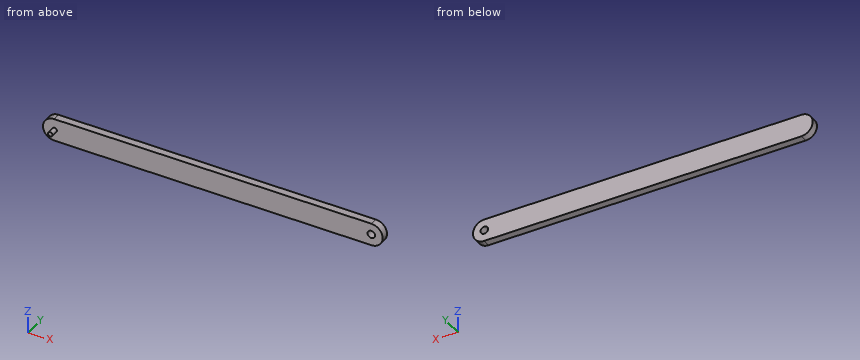
from build123d import *

# Parameters (mm, degrees)
SKETCH1_W           = 114.3
SKETCH1_H           = 7.62
BOSS_EXTRUDE1_DEPTH = 2.54
FILLET1_RADIUS      = 3.81
FILLET1_LENGTH      = 2.54
FILLET4_RADIUS      = 3.81
FILLET4_LENGTH      = 2.54
SKETCH4_R           = 1.27
CUT_EXTRUDE1_DEPTH  = 2.54
SKETCH6_R           = 0.762
BOSS_EXTRUDE3_DEPTH = 2.54


with BuildPart() as part:
    # Sketch1 → Boss-Extrude1 (new body)
    with BuildSketch(Plane(origin=(0, 0, 0), x_dir=(1, 0, 0), z_dir=(0, 1, 0))):
        Rectangle(SKETCH1_W, SKETCH1_H)
    extrude(amount=BOSS_EXTRUDE1_DEPTH)

    # Fillet1: full round fillet: the end face becomes a half cylinder, R = half its width
    fillet1_face = Plane((57.15, 1.27, 0), x_dir=(0, -1, 0), z_dir=(1, 0, 0))  # on the end face: x along it, z out of the body
    fillet1_slab = fillet1_face.offset(-FILLET1_RADIUS / 2) * Box(FILLET1_LENGTH, 2 * FILLET1_RADIUS, FILLET1_RADIUS, mode=Mode.PRIVATE)  # the body's end, R deep
    fillet1_round = Plane((53.34, 1.27, 0), x_dir=(1, 0, 0), z_dir=(0, -1, 0)) * Cylinder(FILLET1_RADIUS, FILLET1_LENGTH, mode=Mode.PRIVATE)  # its axis R under the face
    add(fillet1_slab - fillet1_round, mode=Mode.SUBTRACT)

    # Fillet4: full round fillet: the end face becomes a half cylinder, R = half its width
    fillet4_face = Plane((-57.15, 1.27, 0), x_dir=(0, 1, 0), z_dir=(-1, 0, 0))  # on the end face: x along it, z out of the body
    fillet4_slab = fillet4_face.offset(-FILLET4_RADIUS / 2) * Box(FILLET4_LENGTH, 2 * FILLET4_RADIUS, FILLET4_RADIUS, mode=Mode.PRIVATE)  # the body's end, R deep
    fillet4_round = Plane((-53.34, 1.27, 0), x_dir=(-1, 0, 0), z_dir=(0, 1, 0)) * Cylinder(FILLET4_RADIUS, FILLET4_LENGTH, mode=Mode.PRIVATE)  # its axis R under the face
    add(fillet4_slab - fillet4_round, mode=Mode.SUBTRACT)

    # Sketch4 → Cut-Extrude1 (cut)
    with BuildSketch(Plane(origin=(0, 0, 0), x_dir=(-1, 0, 0), z_dir=(0, -1, 0))):
        with Locations(Location((-53.34, 0, 0), (0, 0, 90))):
            Circle(SKETCH4_R)
    extrude(amount=-CUT_EXTRUDE1_DEPTH, mode=Mode.SUBTRACT)

    # Sketch6 → Boss-Extrude3 (add)
    with BuildSketch(Plane(origin=(0, 0, 0), x_dir=(-1, 0, 0), z_dir=(0, -1, 0))):
        with Locations(Location((53.234546108, 0, 0), (0, 0, 90))):
            Circle(SKETCH6_R)
    extrude(amount=BOSS_EXTRUDE3_DEPTH)


solid = part.part
The listing builds one solid part. Answer for the finished solid, in the listing's coordinates (mm). Coordinates: 2 decimals unless noted, no trailing zeros. Write each loop counter-clockwise with the first axis right and the second up, starting at its lowest first coordinate (ties: lowest second). Pieces come first, ordered by that corner, then holes. Notation, with made-up numbers: M 68,21.25 L 87,21.25 A14 ccw 87,28.25 Z; hole C 48,-29 d2. An arc over 180 degrees is marked long. Write each question's results on one line, items separated by ' | '.
Item 1: The part is cut by section A-A on y = 1.75. Determine the outline of the cut face in (x, z), and give its area (3 significant figures).
Answer below:
outline: M -53.34,-3.81 L 53.34,-3.81 A3.81 ccw 53.34,3.81 L -53.34,3.81 A3.81 ccw Z; hole C 53.34,0 d2.54 | area: 853 mm2
Item 2: Given P1, Ø4, axis at x = 19, z = 0, coming from the -Y side; P2, Ø1.5, axis at y = -2, z = -0.5, coming from the -X side, each flat-ended and moving along its own axis, determine where each tip first touches the part or whether it passes through.
Answer below:
P1: y = 0 | P2: x = -54
Item 3: The part is cut by section B-B on x = 18. Determine the outline of the cut face in (y, z), and give its area (3 significant figures).
Answer below:
outline: M 0,-3.81 L 2.54,-3.81 L 2.54,3.81 L 0,3.81 Z | area: 19.4 mm2
Item 4: Consider probe 1 along X at (y, z) = (1.25, 0); probe 2 along Y at (x, z) = (39.5, 1.75); probe 3 along X at (y, z) = (0.2, 3). Determine where each line is inside the solid, lowest interval first. Write a range as [from, to].
Answer below:
probe 1: [-57.15, 52.07], [54.61, 57.15] | probe 2: [0, 2.54] | probe 3: [-55.69, 55.69]
